from build123d import *

# Parameters (mm, degrees)
SCHIZZO1_R        = 6
ESTRUSIONE1_DEPTH = 37
SCHIZZO3_R        = 4
ESTRUSIONE2_DEPTH = 25
ESTRUSIONE3_START = 25
SCHIZZO4_R        = 4
ESTRUSIONE3_DEPTH = 25
SMUSSO1_SIZE      = 0.5


with BuildPart() as part:
    # Schizzo1 → Estrusione1 (new body)
    with BuildSketch(Plane.XY):
        Circle(SCHIZZO1_R)
    extrude(amount=ESTRUSIONE1_DEPTH)

    # Schizzo3 → Estrusione2 (add)
    with BuildSketch(Plane.XY.offset(37)):
        Circle(SCHIZZO3_R)
    extrude(amount=ESTRUSIONE2_DEPTH)

    # Schizzo4 → Estrusione3 (add)
    with BuildSketch(Plane(origin=(0, 0, 0), x_dir=(-1, 0, 0), z_dir=(0, 0, -1)).offset(ESTRUSIONE3_START)):
        with Locations(Location((0, 0, 0), (0, 0, 180))):
            Circle(SCHIZZO4_R)
    extrude(amount=-ESTRUSIONE3_DEPTH)

    # Smusso1
    smusso1_edges = [part.edges().sort_by_distance(p)[0] for p in [
        (-4, 0, -25),
        (-4, 0, 62),
    ]]
    chamfer(smusso1_edges, length=SMUSSO1_SIZE)


solid = part.part
Work out the finished part from the listing and answer in its coordinate system (mm). A direction names the side the tool comes from. Round coordinates to 2 decimals unless told otherwise and drop trailing zeros. Write each loop counter-clockwise with the first axis right and the second up, starting at its lowest first coordinate (ties: lowest second). Pieces come first, ordered by that corner, then holes. Notation, with made-up numbers: (-19.75, 24) -> (10.25, 24) arc R22 ccw to (10.25, 55) -> close; hole circle Ø5 at (-17.5, 72). An arc over 180 degrees is marked (long way). Answer as CSV lines item,"result". Start each with the question number.
(1) The part is cut by section D-D, the plane z = -19. Give the vertices of the cut face in (x, y), then the cut area to 3 significant figures.
(2) Each of these flat-tipped pins is pushed along its axis until it touches: pin 1 (1 mm diameter, centred on y = 3.5, z = 29.5, fed in from -X); pin 2 (1.5 mm diameter, centred on y = 1, z = 22, fed in from -X); pin 3 (1 mm diameter, centred on x = 3.5, z = 5, fed in from +Y). Where does it stop, or does it pass through?
(3) A tool of negligible diameter and unlimited length cuts with its end or side. For faces 1 (the flat face through (-1.42, -3.92, 0)), 2 (the flat face through (0, 0, -25)), 3 (the cylindrical face through (-0.867, -3.905, 49.078)), from which of +Z, -Z, +X, -X, +Y, -Y can it reach the whole face along a straight path? Write none if from no direction.
(4) The part is cut by section A-A, the plane x = 0. Give the vertices of the cut face in (y, z), then the cut area to 4 significant figures.
(5) The part is cut by section C-C, the plane z = 26. Give the vertices of the cut face in (x, y), then the cut area to 3 significant figures.
(6) Find the intervals of material crossed by probe 1 along Z at (x, y) = (5, 2.75); probe 2 along Y at (x, z) = (-1.5, 10); probe 3 along X at (y, z) = (-5.25, 8), in increasing order.
Output values:
1,outline,"circle Ø8 at (0, 0)"
1,area,"50.3 mm²"
2,pin 1,"stops at x = -5.2"
2,pin 2,"stops at x = -5.99"
2,pin 3,"stops at y = 5.2"
3,face 1,"-Z"
3,face 2,"-Z, +X, -X, +Y, -Y"
3,face 3,"+Z"
4,outline,"(-6, 0) -> (-4, 0) -> (-4, -24.5) -> (-3.5, -25) -> (3.5, -25) -> (4, -24.5) -> (4, 0) -> (6, 0) -> (6, 37) -> (4, 37) -> (4, 61.5) -> (3.5, 62) -> (-3.5, 62) -> (-4, 61.5) -> (-4, 37) -> (-6, 37) -> close"
4,area,"843.5 mm²"
5,outline,"circle Ø12 at (0, 0)"
5,area,"113 mm²"
6,probe 1,"z = 0 to 37"
6,probe 2,"y = -5.81 to 5.81"
6,probe 3,"x = -2.9 to 2.9"
